Geometry: final body of the model. Coordinates: model frame, mm. A direction names the side the tool comes from. Round coordinates to 2 decimals unless told otherwise and drop trailing zeros. Loops run counter-clockwise (first coordinate to the right, second up) from the corner with the lowest first, then second, coordinate; pieces in that order, holes last. Notation, with made-up numbers: (80, 31.25) - (97, 31.25) arc R21 ccw to (97, 63.25) - close; hole circle Ø7 at (-12, 13). An arc over 180 degrees is marked (long way). Return JSON: item names as keys, results as strings. Group by question number.
1. Section C-C on y = 2.25. Return loops of the section in (x, z), and give its area (3 significant figures).
2. Section B-B on x = -5.5. Return loops of the section in (y, z), and give its area (3 significant figures).
3. Section D-D on x = -2.5. Return loops of the section in (y, z), and give its area (4 significant figures).
4. Material intervals for probe 1 along X at (y, z) = (0.5, -7.5); probe 2 along Z at (x, y) = (-3.5, 2.25); probe 3 along X at (y, z) = (0.75, -8.25), sorted ascending.
5. Section A-A on z = 13.5. Return loops of the section in (x, y), and give its area (3 significant figures).
6. First-contact query: pin 1 Ø2 at (x, y) = (2, -0.5) entering from +Z; pin 2 Ø0.8 at (x, y) = (-2.5, 4.5) entering from +Z; pin 3 Ø0.6 at (x, y) = (0, 3) entering from +Z. Flat tips, straight axial feed; report the tip coordinate or a pass-through.
7. Set-up query: faces 4 (the face through (0, 5.5, 11)), 5 (the face through (-3, -1, 1)), 6 (the face through (0, -1, -6)). Return all of +Z, -Z, +X, -X, +Y, -Y with unobstructed straight access to the full face (end or side cutting, diameter ignored); none if empty.
8. Draft query along Y for faces 1 (the face through (1.699, 3.315, -9.021)), 2 (the face through (2.4, 4.5, 7.5)), 3 (the face through (0, 3, -10.5)). Return one class per face: +Y half, -Y half, draft (parallel to the pull), parting line (faces both ways), or undercut.
from build123d import *

# Parameters (mm, degrees)
ESBO_O1_W                = 15
ESBO_O1_H                = 19
ESBO_O1_R                = 1
RESSALTO_EXTRUS_O1_DEPTH = 1.6
ESBO_O3_W                = 4
ESBO_O3_H                = 3
RESSALTO_EXTRUS_O2_DEPTH = 2
FILETE1_R                = 1
ESBO_O4_W                = 8
ESBO_O4_H                = 2.5
RESSALTO_EXTRUS_O3_DEPTH = 2.4
RESSALTO_EXTRUS_O4_DEPTH = 3
CORTE_EXTRUS_O1_START    = -2
ESBO_O6_W                = 1.2
ESBO_O6_H                = 8
CORTE_EXTRUS_O1_DEPTH    = 2
ESBO_O7_W                = 6
ESBO_O7_H                = 14
RESSALTO_EXTRUS_O5_DEPTH = 1.5


with BuildPart() as part:
    # Esboço1 → Ressalto-extrusão1 (new body)
    with BuildSketch(Plane(origin=(0, 0, 0), x_dir=(1, 0, 0), z_dir=(0, 1, 0))):
        Rectangle(ESBO_O1_W, ESBO_O1_H)
        with Locations(Location((-5.5, 7.5, 0), (0, 0, 270))):
            Circle(ESBO_O1_R, mode=Mode.SUBTRACT)
        with Locations(Location((5.5, 7.5, 0), (0, 0, 270))):
            Circle(ESBO_O1_R, mode=Mode.SUBTRACT)
    extrude(amount=RESSALTO_EXTRUS_O1_DEPTH)

    # Esboço3 → Ressalto-extrusão2 (add)
    with BuildSketch(Plane(origin=(0, 1.6, 0), x_dir=(1, 0, 0), z_dir=(0, 1, 0))):
        with Locations((0, 9)):
            Rectangle(ESBO_O3_W, ESBO_O3_H)
    extrude(amount=RESSALTO_EXTRUS_O2_DEPTH)

    # Filete1
    filete1_edges = [part.edges().sort_by_distance(p)[0] for p in [
        (2, 3.6, -9),
        (-2, 3.6, -9),
    ]]
    fillet(filete1_edges, radius=FILETE1_R)

    # Esboço4 → Ressalto-extrusão3 (add)
    with BuildSketch(Plane(origin=(0, 1.6, 0), x_dir=(1, 0, 0), z_dir=(0, 1, 0))):
        with Locations((0, -7.25)):
            Rectangle(ESBO_O4_W, ESBO_O4_H)
    extrude(amount=RESSALTO_EXTRUS_O3_DEPTH)

    # Esboço5 → Ressalto-extrusão4 (add, symmetric)
    with BuildSketch(Plane(origin=(0, 0, 0), x_dir=(0, 0, -1), z_dir=(1, 0, 0))):
        with BuildLine():
            Line((-7.5, 4), (-7.5, 5))
            ThreePointArc((-7.5, 5), (-7.646446609, 5.353553391), (-8, 5.5))
            Line((-8, 5.5), (-15, 5.5))
            Line((-15, 5.5), (-15, 6))
            Line((-15, 6), (-7.5, 6))
            ThreePointArc((-7.5, 6), (-7.146446609, 5.853553391), (-7, 5.5))
            Line((-7, 5.5), (-7, 4))
            Line((-7, 4), (-7.5, 4))
        make_face()
    extrude(amount=RESSALTO_EXTRUS_O4_DEPTH, both=True)

    # Esboço6 → Corte-extrusão1 (cut)
    with BuildSketch(Plane(origin=(0, 6, 0), x_dir=(1, 0, 0), z_dir=(0, 1, 0)).offset(CORTE_EXTRUS_O1_START)):
        with Locations((-1.2, -11)):
            Rectangle(ESBO_O6_W, ESBO_O6_H)
        with Locations((1.2, -11)):
            Rectangle(ESBO_O6_W, ESBO_O6_H)
    extrude(amount=CORTE_EXTRUS_O1_DEPTH, mode=Mode.SUBTRACT)

    # Esboço7 → Ressalto-extrusão5 (add)
    with BuildSketch(Plane.XZ):
        with Locations((0, 1)):
            Rectangle(ESBO_O7_W, ESBO_O7_H)
    extrude(amount=RESSALTO_EXTRUS_O5_DEPTH)


solid = part.part
Taken from the geometry:
{
 "1": {"outline": "(-4, 6) - (4, 6) - (4, 8.5) - (-4, 8.5) - close; (-2, -10.5) - (2, -10.5) - (2, -7.5) - (-2, -7.5) - close", "area": "32.0 mm2"},
 "2": {"outline": "(0, -9.5) - (1.6, -9.5) - (1.6, -8.5) - (0, -8.5) - close; (0, -6.5) - (1.6, -6.5) - (1.6, 9.5) - (0, 9.5) - close", "area": "27.2 mm2"},
 "3": {"outline": "(-1.5, -6) - (0, -6) - (0, -9.5) - (1.6, -9.5) - (1.6, 6) - (4, 6) - (4, 7) - (5.5, 7) arc R0.5 ccw to (6, 7.5) - (6, 15) - (5.5, 15) - (5.5, 8) arc R0.5 cw to (5, 7.5) - (4, 7.5) - (4, 8.5) - (1.6, 8.5) - (1.6, 9.5) - (0, 9.5) - (0, 8) - (-1.5, 8) - close", "area": "62.15 mm2"},
 "4": {"probe 1": "-7.5 to -6.5, -4.5 to 4.5, 6.5 to 7.5", "probe 2": "6 to 8.5", "probe 3": "-7.5 to -6.16, -4.84 to 4.84, 6.16 to 7.5"},
 "5": {"outline": "(-3, 5.5) - (-1.8, 5.5) - (-1.8, 6) - (-3, 6) - close; (-0.6, 5.5) - (0.6, 5.5) - (0.6, 6) - (-0.6, 6) - close; (1.8, 5.5) - (3, 5.5) - (3, 6) - (1.8, 6) - close", "area": "1.80 mm2"},
 "6": {"pin 1": "z = 9.5", "pin 2": "z = 7.5", "pin 3": "z = 8.5"},
 "7": {"face 4": "+Z, +X, -X", "face 5": "+Z, -Z, -X, -Y", "face 6": "-Z, +X, -X, -Y"},
 "8": {"face 1": "+Y half", "face 2": "undercut", "face 3": "draft"}
}
